Source: three-view drawing plus pictorial views. Frame: mm from the lowest corner of the part. A direction names the side the tool comes from. Round coordinates to 2 decimals unless told otherwise and drop trailing zeros. Loops run counter-clockwise (first coordinate to the right, second up) from the corner with the lowest first, then second, coordinate; pieces in that order, holes last. Notation, with made-up numbers: (19.25, -14.75) -> (55.25, -14.75) arc R18 ccw to (55.25, 18.25) -> close; hole circle Ø6 at (4, -8). An arc over 180 degrees is marked (long way). Answer as a JSON object with one key per item and string values. Group by question number.
Item 1: Draft query along X for the marked faces 4, 5, 6 and 7. Return one class per face: released by +X, released by -X, zero draft, split by the parting line, or undercut.
Item 2: Section query C-C on z = 15. Return loops of the section in (x, y), and give its area (3 significant figures).
Item 3: Set-up query: the marked faces 1, 2 and 3. Return all of +Z, -Z, +X, -X, +Y, -Y with unobstructed straight access to the full face (end or side cutting, diameter ignored); none if empty.
Item 4: Pin query (flat end, axial travel): pin 1 (12 mm diameter, centred on x = 15.5, z = 17, fed in from -Y); pin 2 (2 mm diameter, centred on y = 30, z = 6.5, fed in from +X); pin 3 (4 mm diameter, centred on y = 38.5, z = 10, fed in from -X). Return the tip coordinate at first contact, or that it passes through.
Item 5: Material intervals for line 1 (Y direction, x = 21.5, z = 3.3); line 2 (Y direction, x = 21.5, z = 4.2); line 3 (Z direction, x = 18.5, y = 41.5), sorted ascending. Write a range as [from, to].
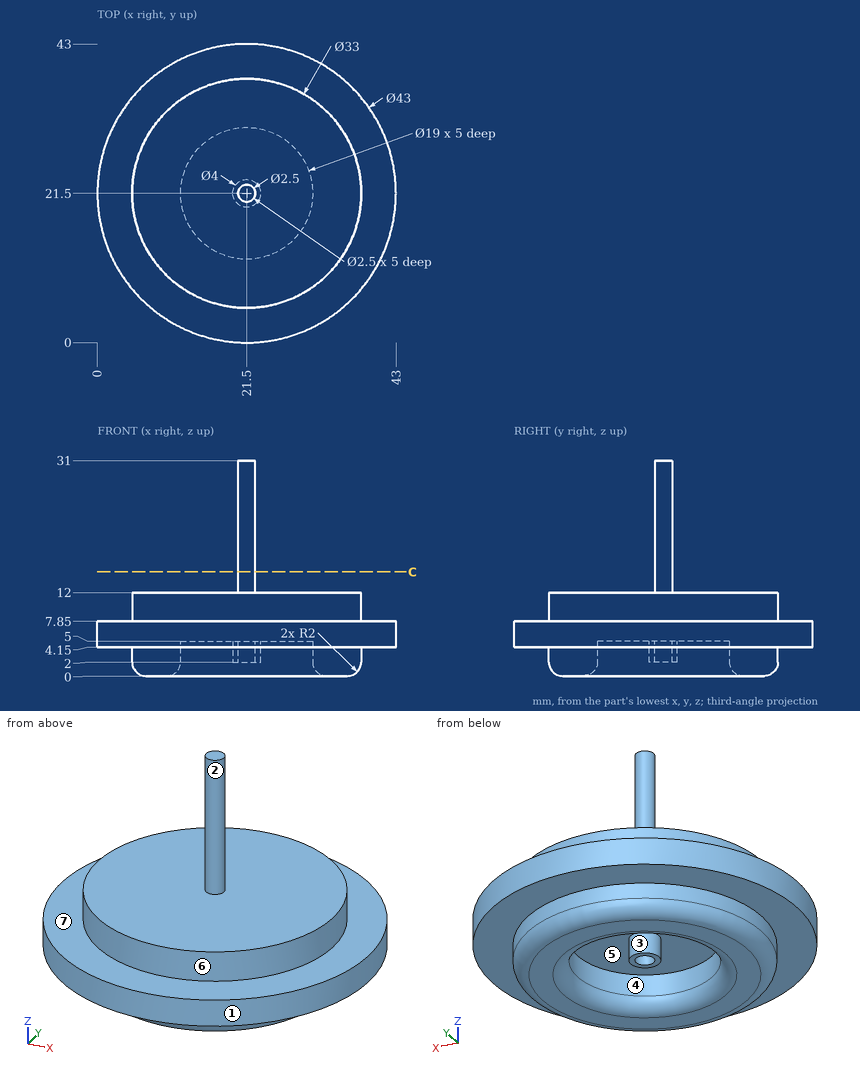
Solved:
{
 "1": {"face 4": "undercut", "face 5": "undercut", "face 6": "split by the parting line", "face 7": "zero draft"},
 "2": {"outline": "circle Ø2.5 at (21.5, 21.5)", "area": "4.91 mm²"},
 "3": {"face 1": "+Z, -Z", "face 2": "+Z", "face 3": "-Z"},
 "4": {"pin 1": "y = 5.22", "pin 2": "x = 41.65", "pin 3": "x = 14.63"},
 "5": {"line 1": "[5, 12], [19.5, 20.25], [22.75, 23.5], [31, 38]", "line 2": "[0, 12], [19.5, 20.25], [22.75, 23.5], [31, 43]", "line 3": "[4.15, 7.85]"}
}
